```python
from build123d import *

# Parameters (mm, degrees)
SKETCH1_R           = 5
BOSS_EXTRUDE1_DEPTH = 15


with BuildPart() as part:
    # Sketch1 → Boss-Extrude1 (new body)
    with BuildSketch(Plane.XY):
        Polygon((0, 0), (0, 12.5), (-15, 12.5), (-15, 27.5), (0, 27.5), (0, 52.5), (-15, 52.5), (-15, 67.5), (0, 67.5), (0, 80), (384, 80), (384, 67.5), (399, 67.5), (399, 52.5), (384, 52.5), (384, 27.5), (399, 27.5), (399, 12.5), (384, 12.5), (384, 0), (303, 0), (303, 15), (283, 15), (283, 0), (202, 0), (202, 15), (182, 15), (182, 0), (101, 0), (101, 15), (81, 15), (81, 0), align=None)
        with Locations((17.3, 30)):
            Circle(SKETCH1_R, mode=Mode.SUBTRACT)
        with Locations(Location((366.7, 30, 0), (0, 0, 180))):  # turned: the seam where the file's is
            Circle(SKETCH1_R, mode=Mode.SUBTRACT)
    extrude(amount=BOSS_EXTRUDE1_DEPTH)


solid = part.part
```
Verification items for the finished model (mm, model axes). A direction names the side the tool comes from. Coordinates: 2 decimals unless noted, no trailing zeros. Write each loop counter-clockwise with the first axis right and the second up, starting at its lowest first coordinate (ties: lowest second). Pieces come first, ordered by that corner, then holes. Notation, with made-up numbers: M 75.25,58 L 104.25,58 A15 ccw 104.25,67 Z; hole C 45,74 d9. An arc over 180 degrees is marked long. One line per item, written item: value.
Item 1: Section check D-D, the plane y = 73. Record the boundary of the cut face in (x, z).
Check sheet entries:
outline: M 0,0 L 384,0 L 384,15 L 0,15 Z
Item 2: Gauge pin test, flat ends, axial feed: pin 1 Ø4.5 at (y, z) = (44, 4.5) entering from +X; pin 2 Ø4.5 at (x, z) = (-10, 9) entering from +Y; pin 3 Ø4 at (x, z) = (168, 10) entering from -Y; pin 4 Ø8 at (x, y) = (366.7, 30) entering from -Z. Record the tip position at first contact, or that the pin passes through.
Check sheet entries:
pin 1: stops at x = 384
pin 2: stops at y = 67.5
pin 3: stops at y = 0
pin 4: passes through
Item 3: Section check A-A, the plane y = 5.5. Record the boundary of the cut face in (x, z), plus the area to 3 significant figures.
Check sheet entries:
outline: M 0,0 L 81,0 L 81,15 L 0,15 Z; M 101,0 L 182,0 L 182,15 L 101,15 Z; M 202,0 L 283,0 L 283,15 L 202,15 Z; M 303,0 L 384,0 L 384,15 L 303,15 Z
area: 4,860 mm^2
Item 4: Section check C-C, the plane x = 366.7. Record the boundary of the cut face in (y, z).
Check sheet entries:
outline: M 0,0 L 25,0 L 25,15 L 0,15 Z; M 35,0 L 80,0 L 80,15 L 35,15 Z
Item 5: Scan lines: line 1 along X through (y, z) = (13.5, 14); line 2 along X through (y, z) = (3, 3.75); line 3 along Y through (x, z) = (17.3, 6). Record each from-to range of solid material in increasing order.
Check sheet entries:
line 1: x = -15 to 81, 101 to 182, 202 to 283, 303 to 399
line 2: x = 0 to 81, 101 to 182, 202 to 283, 303 to 384
line 3: y = 0 to 25, 35 to 80
Item 6: Section check B-B, the plane z = 11.75. State how many separate pieces and enclosed holes the cut face has, plus the area to 3 significant figures.
Check sheet entries:
separate pieces: 1
enclosed holes: 2
area: 30,600 mm^2
Item 7: Mould release check, pull along Y, two halves, no side actions. Record for faces 6 (the flat face through (41, 0, 7)), 7 (the flat face through (-8, 27.5, 7)), 8 (the flat face through (-15, 60, 7)): pulls with the +Y half, pulls with the -Y half, needs draft (parallel to the pull), parting line crosses it, or undercut.
Check sheet entries:
face 6: pulls with the -Y half
face 7: undercut
face 8: needs draft
Item 8: Access from +Z, -Z, +X, -X, +Y, -Y to the whole of each face (thin tool, end or side, straight path). Record for faces 1 (the flat face through (0, 74, 7)), 2 (the flat face through (391, 67.5, 7)), 3 (the flat face through (-7, 52.5, 7)), 4 (the flat face through (391, 27.5, 7)), 5 (the flat face through (182, 8, 7)).
Check sheet entries:
face 1: +Z, -Z, -X, +Y
face 2: +Z, -Z, +X, +Y
face 3: +Z, -Z, -X
face 4: +Z, -Z, +X
face 5: +Z, -Z, -Y
